Part model, mm, in its own coordinate system. A direction names the side the tool comes from. Coordinates: 2 decimals unless noted, no trailing zeros. Write each loop counter-clockwise with the first axis right and the second up, starting at its lowest first coordinate (ties: lowest second). Pieces come first, ordered by that corner, then holes. Notation, with made-up numbers: M -0.75,-8 L 39.25,-8 A12 cw 39.25,13 Z; hole C 72.5,-21 d8. An arc over 180 degrees is marked long. Use a Markdown table: item, result. Add a question column.
Q1. Pin check, flat tips, straight feed: pin 1 Ø5 at (y, z) = (6.5, 85.5) entering from -X; pin 2 Ø9 at (x, y) = (-15, 14.5) entering from +Z; pin 3 Ø10 at (x, z) = (-17.5, 101.5) entering from +Y; pin 4 Ø4 at (x, y) = (-24, 3) entering from -Z. Stop position of each tip, or through.
Q2. Slice it at D-D on y = 6.25. Write the cut outline in (x, z).
Q3. Slice it at C-C on z = 83. Write the cut outline in (x, y).
Q4. Tool access for faces 1 (the cylindrical face through (-7.2, 9.1, 105)), 2 (the cylindrical face through (-11.4, 19.43, 98.08)), 3 (the flat face through (-8, 0, 86)), 4 (the cylindrical face through (-25.52, 2.4, 82.89)), 5 (the flat face through (-12, 10, 98)): list every direction of +Z, -Z, +X, -X, +Y, -Y with a clear straight run to the whole face (end or side of a thin tool).
Q5. Wall check: L1, parallel to Y at x = -15.5, z = 74.35; L2, parallel to Y at x = -3.5, z = 82; L3, parallel to Z at x = -5, y = 15.75. Give the ranges that are in metal, low to high. Write a range as from..to.
Q6. Slice it at B-B on x = -15.5. Write the cut outline in (y, z), then the cut area to 3 significant figures.
Q7. Mould opens along Y. For faces 6 (the flat face through (-14.8, 9.9, 91)), 7 (the cylindrical face through (-4.93, 19.43, 105.4)), 8 (the cylindrical face through (-15.9, 19.5, 83.3)) say: released by +Y, released by -Y, zero draft, split by the parting line, or undercut.
Q8. Slice it at A-A on y = 10. Write the cut outline in (x, z), then the cut area to 3 significant figures.
Autodesk Inventor part; units mm, degrees
ref_plane "Work Plane1" through (-21, 0, 91.5) normal (0, 0, 1) x (1, 0, 0)
ref_plane "Work Plane2" through (0, 10, 0) normal (0, 1, 0) x (-1, 0, 0)
ref_plane "YZ Plane" through (0, 0, 0) normal (1, 0, 0) x (0, 1, 0)
sketch "Sketch1" plane through (0, 0, 0) normal (0, 1, 0) x (-1, 0, 0)
  line L0 (0, -106) -> (0, 94)
  line L1 (0, -106) -> (21, -106) construction
  line L2 (30, -97) -> (30, -97) construction
  line L3 (0, -106) -> (12, -106) construction
  line L4 (21, -88) -> (12, -88) construction
  line L5 (12, -88) -> (12, -86)
  line L6 (12, -106) -> (21, -106)
  line L7 (30, -88) -> (21, -88) construction
  line L8 (30, -88) -> (30, -106) construction
  arc A0 (21, -106) -> (30, -97) centre (21, -97) ccw
  arc A1 (30, -97) -> (21, -88) centre (21, -97) ccw
  line L9 (21, -106) -> (30, -106) construction
  line L10 (21, -88) -> (12, -88)
  line L11 (12, -68) -> (12, -66)
  arc A2 (21, -86) -> (30, -77) centre (21, -77) ccw
  arc A3 (30, -77) -> (21, -68) centre (21, -77) ccw
  line L12 (0, -86) -> (21, -86) construction
  line L13 (21, -68) -> (12, -68) construction
  line L14 (21, -68) -> (12, -68)
  line L15 (12, -86) -> (21, -86)
  line L16 (12, -48) -> (12, -46)
  arc A4 (21, -66) -> (30, -57) centre (21, -57) ccw
  arc A5 (30, -57) -> (21, -48) centre (21, -57) ccw
  line L17 (0, -66) -> (21, -66) construction
  line L18 (21, -48) -> (12, -48) construction
  line L19 (21, -48) -> (12, -48)
  line L20 (12, -66) -> (21, -66)
  line L21 (12, -28) -> (12, -26)
  arc A6 (21, -46) -> (30, -37) centre (21, -37) ccw
  arc A7 (30, -37) -> (21, -28) centre (21, -37) ccw
  line L22 (0, -46) -> (21, -46) construction
  line L23 (21, -28) -> (12, -28) construction
  line L24 (21, -28) -> (12, -28)
  line L25 (12, -46) -> (21, -46)
  line L26 (12, -8) -> (12, -6)
  arc A8 (21, -26) -> (30, -17) centre (21, -17) ccw
  arc A9 (30, -17) -> (21, -8) centre (21, -17) ccw
  line L27 (0, -26) -> (21, -26) construction
  line L28 (21, -8) -> (12, -8) construction
  line L29 (21, -8) -> (12, -8)
  line L30 (12, -26) -> (21, -26)
  line L31 (12, 12) -> (12, 14)
  arc A10 (21, -6) -> (30, 3) centre (21, 3) ccw
  arc A11 (30, 3) -> (21, 12) centre (21, 3) ccw
  line L32 (0, -6) -> (21, -6) construction
  line L33 (21, 12) -> (12, 12) construction
  line L34 (21, 12) -> (12, 12)
  line L35 (12, -6) -> (21, -6)
  line L36 (12, 32) -> (12, 34)
  arc A12 (21, 14) -> (30, 23) centre (21, 23) ccw
  arc A13 (30, 23) -> (21, 32) centre (21, 23) ccw
  line L37 (0, 14) -> (21, 14) construction
  line L38 (21, 32) -> (12, 32) construction
  line L39 (21, 32) -> (12, 32)
  line L40 (12, 14) -> (21, 14)
  line L41 (12, 52) -> (12, 54)
  arc A14 (21, 34) -> (30, 43) centre (21, 43) ccw
  arc A15 (30, 43) -> (21, 52) centre (21, 43) ccw
  line L42 (0, 34) -> (21, 34) construction
  line L43 (21, 52) -> (12, 52) construction
  line L44 (21, 52) -> (12, 52)
  line L45 (12, 34) -> (21, 34)
  line L46 (12, 72) -> (12, 74)
  arc A16 (21, 54) -> (30, 63) centre (21, 63) ccw
  arc A17 (30, 63) -> (21, 72) centre (21, 63) ccw
  line L47 (0, 54) -> (21, 54) construction
  line L48 (21, 72) -> (12, 72) construction
  line L49 (21, 72) -> (12, 72)
  line L50 (12, 54) -> (21, 54)
  line L51 (12, 92) -> (12, 94)
  arc A18 (21, 74) -> (30, 83) centre (21, 83) ccw
  arc A19 (30, 83) -> (21, 92) centre (21, 83) ccw
  line L52 (0, 74) -> (21, 74) construction
  line L53 (21, 92) -> (12, 92) construction
  line L54 (21, 92) -> (12, 92)
  line L55 (12, 74) -> (21, 74)
  line L56 (0, 94) -> (0, 106)
  line L57 (0, 106) -> (6, 106)
  line L58 (12, 100) -> (12, 94)
  line L59 (12, -106) -> (0, -106)
  line L60 (12, 100) -> (12, 106)
  line L61 (12, 106) -> (6, 106)
  line L62 (0, -106) -> (64, -106)
  line L63 (64, -106) -> (64, 74)
  line L64 (64, 74) -> (0, 74)
  line L65 (0, 74) -> (0, -106)
  point P0 (0, 0)
  point P1 (30, -86)
  point P2 (30, -68)
  point P3 (30, -66)
  point P4 (30, -48)
  point P5 (30, -46)
  point P6 (30, -28)
  point P7 (30, -26)
  point P8 (30, -8)
  point P9 (30, -6)
  point P10 (30, 12)
  point P11 (30, 14)
  point P12 (30, 32)
  point P13 (30, 34)
  point P14 (30, 52)
  point P15 (30, 54)
  point P16 (30, 72)
  point P17 (30, 74)
  point P18 (30, 92)
  point P19 (30, -97)
  point P20 (21, 74)
  point P21 (0, 74)
  dimension "d0" = 94
  dimension "d1" = 110.1635
  dimension "d2" = 18
  dimension "d3" = 106.6771
  dimension "d4" = 2
  dimension "d5" = 9
  dimension "d6" = 9
  dimension "d11" = 20
  dimension "d16" = 12
  dimension "d17" = 12
  dimension "d60" = 64
extrude "Extrusion1" add sketch "Sketch1" along normal blind 20 contours L0 L64 L46 L49 A17 A16 L50 L41 L44 A15 A14 L45 L36 L39 A13 A12 L40 L31 L34 A11 A10 L35 L26 L29 A9 A8 L30 L21 L24 A7 A6 L25 L16 L19 A5 A4 L20 L11 L14 A3 A2 L15 L5 L10 A1 A0 L6 L59 | L0 L56 L57 L61 L60 L58 L51 L54 A19 A18 L55 L64
sketch "Sketch2" plane through (0, 0, -106) normal (0, 0, -1) x (-1, 0, 0)
  line L0 (30, 20) -> (21, 20) construction
  line L1 (21, 20) -> (0, 20)
  line L2 (0, 20) -> (0, 0)
  line L3 (0, 0) -> (21, 0)
  line L4 (30, 9) -> (30, 11)
  line L5 (30, 20) -> (0, 0) construction
  arc A0 (30, 11) -> (21, 20) centre (21, 11) ccw
  arc A1 (21, 0) -> (30, 9) centre (21, 9) ccw
  line L6 (5.5, -4) -> (24.5, -4)
  line L7 (24.5, -4) -> (24.5, 24)
  line L8 (24.5, 24) -> (5.5, 24)
  line L9 (5.5, 24) -> (5.5, -4)
  line L10 (5.5, -4) -> (24.5, 24) construction
  line L11 (24.5, -4) -> (5.5, 24) construction
  line L12 (24.5, 24) -> (37.5, 24)
  line L13 (37.5, 24) -> (37.5, 0)
  line L14 (37.5, 0) -> (24.5, -4)
  point P0 (0, 0)
  point P1 (30, 0)
  point P2 (15, 10)
  point P3 (5.5, 0)
  point P4 (5.5, 20)
  dimension "d21" = 30
  dimension "d22" = 20
  dimension "d23" = 9
  dimension "d24" = 9
  dimension "d25" = 19
  dimension "d26" = 28
  dimension "d65" = 13
extrude "Extrusion2" cut sketch "Sketch2" against normal blind 200 contours L1 L9 L8 L7 A0 | L7 L12 L13 L14 A1 L4 A0 | L3 A1 L7 L6 L9
shell "Shell2" thickness 1 removed faces 1 at (-8, 6.6667, 106)
sketch "Sketch7" plane through (-12, 0, 106) normal (0, 0, 1) x (1, 0, 0)
  line L0 (0, 20) -> (12, 20)
  line L1 (0, 0) -> (12, 0)
  line L2 (12, 0) -> (12, 20)
  line L3 (12, 20) -> (0, 20)
  line L4 (0, 20) -> (0, 0)
  circle A0 centre (6, 10) radius 1.5
  point P0 (12, 0)
  dimension "d46" = 3
  dimension "d66" = 6
  dimension "d67" = 10
extrude "Extrusion5" add sketch "Sketch7" against normal blind 14 contours L0 L2 L1 L4 | A0
fillet "Fillet2" radius 2 5 edges at (-12, 20, 99) (-12, 10, 106) (-12, 0, 99) (-6, 0, 106) (-6, 20, 106)
extrude "Extrusion6" cut sketch "Sketch7" against normal blind 2 contours A0
sketch "Sketch8" plane through (0, 0, 0) normal (1, 0, 0) x (0, 1, 0)
  line L0 (0, -88) -> (20, -88)
  line L1 (0, -86) -> (20, -86)
  line L2 (0, 9) -> (20, 9)
  line L3 (20, 9) -> (20, 10)
  line L4 (20, 10) -> (0, 10)
  line L5 (0, 10) -> (0, 9)
  line L6 (0, 19) -> (20, 19)
  line L7 (20, 20) -> (0, 20)
  line L8 (20, 19) -> (20, 20)
  line L9 (0, 20) -> (0, 19)
  line L10 (0, 29) -> (20, 29)
  line L11 (20, 30) -> (0, 30)
  line L12 (20, 29) -> (20, 30)
  line L13 (0, 30) -> (0, 29)
  line L14 (0, 39) -> (20, 39)
  line L15 (20, 40) -> (0, 40)
  line L16 (20, 39) -> (20, 40)
  line L17 (0, 40) -> (0, 39)
  line L18 (0, 49) -> (20, 49)
  line L19 (20, 50) -> (0, 50)
  line L20 (20, 49) -> (20, 50)
  line L21 (0, 50) -> (0, 49)
  line L22 (0, 59) -> (20, 59)
  line L23 (20, 60) -> (0, 60)
  line L24 (20, 59) -> (20, 60)
  line L25 (0, 60) -> (0, 59)
  line L26 (0, 69) -> (20, 69)
  line L27 (20, 70) -> (0, 70)
  line L28 (20, 69) -> (20, 70)
  line L29 (0, 70) -> (0, 69)
  line L30 (0, 79) -> (20, 79)
  line L31 (20, 80) -> (0, 80)
  line L32 (20, 79) -> (20, 80)
  line L33 (0, 80) -> (0, 79)
  line L34 (0, 89) -> (20, 89)
  line L35 (20, 90) -> (0, 90)
  line L36 (20, 89) -> (20, 90)
  line L37 (0, 90) -> (0, 89)
  point P0 (0, 0)
  dimension "d51" = 10
extrude "Extrusion7" [suppressed]
ref_plane "Work Plane1" through (-21, 0, 91.5) normal (0, 0, 1) x (1, 0, 0)
sketch "Sketch4" plane through (-21, 0, 91.5) normal (0, 0, 1) x (1, 0, 0)
  line L0 (0, 0) -> (0, 20)
  line L1 (0, 0) -> (12, 20) construction
  circle A0 centre (6, 10) radius 2 construction
  line L2 (5, 6.5) -> (1, 6.5)
  line L3 (1, 6.5) -> (1, 13.5)
  line L4 (1, 13.5) -> (5, 13.5)
  line L5 (5, 13.5) -> (5, 6.5)
  line L6 (5, 6.5) -> (1, 13.5) construction
  line L7 (1, 6.5) -> (5, 13.5) construction
  point P0 (21, 0)
  point P1 (3, 10)
  point P2 (1, 10)
  point P3 (5, 8.2679)
  dimension "d31" = 4
  dimension "d58" = 4
  dimension "d59" = 7
extrude "Extrusion3" [suppressed]
extrude "Extrusion8" cut sketch "Sketch1" along normal blind 20 contours L0 L64 L46 L49 A17 A16 L50 L41 L44 A15 A14 L45 L36 L39 A13 A12 L40 L31 L34 A11 A10 L35 L26 L29 A9 A8 L30 L21 L24 A7 A6 L25 L16 L19 A5 A4 L20 L11 L14 A3 A2 L15 L5 L10 A1 A0 L6 L59 | L55 L64 L63 L62 A0 A1 L10 L5 L15 A2 A3 L14 L11 L20 A4 A5 L19 L16 L25 A6 A7 L24 L21 L30 A8 A9 L29 L26 L35 A10 A11 L34 L31 L40 A12 A13 L39 L36 L45 A14 A15 L44 L41 L50 A16 A17 L49 L46
sketch "Sketch9" plane through (0, 0, 74) normal (0, 0, -1) x (-1, 0, 0)
  line L0 (11, 19) -> (1, 19)
  line L1 (11, 19) -> (0, 19)
  line L2 (0, 19) -> (0, 0)
  line L3 (0, 0) -> (11, 0)
  line L4 (11, 0) -> (11, 19)
extrude "Extrusion9" add sketch "Sketch9" against normal blind 1
ref_plane "Work Plane2" through (0, 10, 0) normal (0, 1, 0) x (-1, 0, 0)
sketch "Sketch10" plane through (0, 20, 0) normal (0, 1, 0) x (1, 0, 0)
  line L0 (-10, -104) -> (-10, -92) construction
  line L1 (-21, -92) -> (-21, -74) construction
  line L2 (-10, -92) -> (-21, -74) construction
  circle A0 centre (-15.5, -83) radius 0.5
  point P0 (0, 0)
  dimension "d68" = 1
extrude "Extrusion10" cut sketch "Sketch10" against normal through all
sketch "Sketch11" plane through (-21, 0, 92) normal (0, 0, 1) x (1, 0, 0)
  line L0 (0, 0) -> (11, 0) construction
  line L1 (11, 18) -> (11, 20) construction
  line L2 (0, 0) -> (11, 20) construction
  circle A0 centre (5.5, 10) radius 0.5
  point P0 (21, 0)
  dimension "d71" = 1
extrude "Extrusion11" cut sketch "Sketch11" against normal through all
sketch "Sketch6" plane through (0, 10, 0) normal (0, 1, 0) x (-1, 0, 0)
  line L0 (40.7593, 109.726) -> (-19.2407, 109.726)
  line L1 (-19.2407, 109.726) -> (-19.2407, -3.5286)
  line L2 (-19.2407, -3.5286) -> (40.7593, -3.5286)
  line L3 (40.7593, -3.5286) -> (40.7593, 109.726)
  point P0 (0, 0)
  dimension "d36" = 113.2546
  dimension "d37" = 60
properties part number "3D_print_actuator"
Recorded:
| question | item | result |
|---|---|---|
| 1 | pin 1 | x = -29.97 |
| 1 | pin 2 | z = 105.94 |
| 1 | pin 3 | through |
| 1 | pin 4 | z = 74.06 |
| 2 | outline | M -29.57,80.25 A9 ccw -21,74 L 0,74 L 0,106 L -10,106 A2 ccw -12,104 L -12,92 L -21,92 A9 ccw -29.57,85.75 Z; hole M -28.51,80.25 A8 ccw -21,75 L -1,75 L -1,92 L -11,92 L -11,91 L -21,91 A8 ccw -28.51,85.75 Z |
| 3 | outline | M -30,9 A9 ccw -21,0 L -16,0 L -16,1 L -21,1 A8 cw -29,9 L -29,11 A8 cw -21,19 L -16,19 L -16,20 L -21,20 A9 ccw -30,11 Z; M -15,0 L 0,0 L 0,20 L -15,20 L -15,19 L -1,19 L -1,1 L -15,1 Z |
| 4 | face 1 | +Z |
| 4 | face 2 | +Z, -X, +Y |
| 4 | face 3 | +Z, -Z, +X, -X, -Y |
| 4 | face 4 | none |
| 4 | face 5 | +Z, -X, +Y, -Y |
| 5 | L1 | 0..9.5, 10.5..20 |
| 5 | L2 | 0..1, 19..20 |
| 5 | L3 | 74..75, 92..106 |
| 6 | outline | M 0,74 L 9.5,74 L 9.5,75 L 1,75 L 1,82.5 L 0,82.5 Z; M 0,83.5 L 1,83.5 L 1,91 L 9.5,91 L 9.5,92 L 0,92 Z; M 10.5,74 L 20,74 L 20,82.5 L 19,82.5 L 19,75 L 10.5,75 Z; M 10.5,91 L 19,91 L 19,83.5 L 20,83.5 L 20,92 L 10.5,92 Z |
| 6 | area | 68.0 mm² |
| 7 | face 6 | undercut |
| 7 | face 7 | released by +Y |
| 7 | face 8 | zero draft |
| 8 | outline | M -21,74 L -16,74 L -16,75 L -21,75 A8 cw -21,91 L -16,91 L -16,92 L -21,92 A9 ccw Z; M -15,74 L 0,74 L 0,106 L -4.5,106 L -4.5,104 L -7.5,104 L -7.5,106 L -10,106 A2 ccw -12,104 L -12,92 L -15,92 L -15,91 L -11,91 L -11,92 L -1,92 L -1,75 L -15,75 Z |
| 8 | area | 234 mm² |
